```python
from build123d import *

# Parameters (mm, degrees)
F0_R     = 3
F1_DEPTH = 25
F2_DEPTH = 2
F3_DEPTH = 15
F4_SIZE2 = 1
F4_SIZE  = 2
F5_SIZE2 = 2
F5_SIZE  = 1


with BuildPart() as f1:
    # F0 (on Front) → F1 (new body)
    with BuildSketch(Plane.XZ):
        Circle(F0_R)
    extrude(amount=F1_DEPTH)

    # F0 (on Front) → F2 (join)
    with BuildSketch(Plane.XZ):
        with BuildLine():
            ThreePointArc((1.9364916731, -3.5), (3.4457195687, -2.0315060063), (4, 0))
            ThreePointArc((4, 0), (-2.0315060063, 3.4457195687), (-1.9364916731, -3.5))
            Line((-1.9364916731, -3.5), (1.9364916731, -3.5))
        make_face()
        Circle(F0_R, mode=Mode.SUBTRACT)
    extrude(amount=F2_DEPTH)

    # F0 (on Front) → F3 (join)
    with BuildSketch(Plane.XZ):
        Circle(F0_R)
    extrude(amount=-F3_DEPTH)

    # F4
    f4_edges = [f1.edges().sort_by_distance(p)[0] for p in [
        (-3, 15, 0),
    ]]
    f4_side = f1.faces().sort_by_distance((-3, 7.5, 0))[0]
    chamfer(f4_edges, length=F4_SIZE, length2=F4_SIZE2, reference=f4_side)

    # F5
    f5_edges = [f1.edges().sort_by_distance(p)[0] for p in [
        (-3, -25, 0),
    ]]
    f5_side = f1.faces().sort_by_distance((0, -25, 0))[0]
    chamfer(f5_edges, length=F5_SIZE, length2=F5_SIZE2, reference=f5_side)


solid = f1.part
```
The listing builds one solid part. Answer for the finished solid, in the listing's coordinates (mm). A direction names the side the tool comes from. Give positions to 0.01 mm unless a question says otherwise; leave off trailing zeros. Order: outer loops, then holes, each group sorted by start corner. A loop starts at its lowest first (then second) coordinate and runs counter-clockwise, first axis right, second up. Notation, with made-up numbers: (49.25, -18) - (63.25, -18) arc R16 ccw to (63.25, 4) - close; hole circle Ø7 at (-3, 14). An arc over 180 degrees is marked (long way). Answer in a Markdown table with one row per item. Add a question column.
Q1. The part is cut by section B-B (y = 12.5). Determine the outline of the cut face in (x, z), then the cut area to 3 significant figures.
Q2. Find the intervals of material crossed by line 1 along Y through (x, z) = (-3, 1); line 2 along Z through (x, y) = (0.25, -21); line 3 along X through (y, z) = (-6.5, -1.25), in increasing order. Write a range as [from, to].
Q3. The part is cut by section A-A (x = 0). Determine the outline of the cut face in (y, z), then the cut area to 3 significant figures.
Q4. Which of the six approach directions +Z, -Z, +X, -X, +Y, -Y give full straight-line access (tool end or side, diameter ignored) to faces 1 (the flat face through (1, 0, 3)), 2 (the flat face through (1, -2, 3)), 3 (the flat face through (0, 15, 0))?
Q5. Given P1, Ø1, axis at x = 2.5, z = -2.5, coming from the +Y side; P2, Ø1, axis at x = -0.5, y = -18, coming from the +Z side; P3, Ø1, axis at x = 2.5, y = -10.5, coming from the -Z side, each flat-ended and moving along its own axis, determine where each tip first touches the part or whether it passes through.
Determined:
| question | item | result |
|---|---|---|
| 1 | outline | circle Ø6 at (0, 0) |
| 1 | area | 28.3 mm² |
| 2 | line 1 | y = [-2, 0] |
| 2 | line 2 | z = [-2.99, 2.99] |
| 2 | line 3 | x = [-2.73, 2.73] |
| 3 | outline | (-25, -2) - (-23, -3) - (-2, -3) - (-2, -3.5) - (0, -3.5) - (0, -3) - (13, -3) - (15, -2) - (15, 2) - (13, 3) - (0, 3) - (0, 4) - (-2, 4) - (-2, 3) - (-23, 3) - (-25, 2) - close |
| 3 | area | 239 mm² |
| 4 | face 1 | +Y |
| 4 | face 2 | -Y |
| 4 | face 3 | +Z, -Z, +X, -X, +Y |
| 5 | P1 | stops at y = 0 |
| 5 | P2 | stops at z = 3 |
| 5 | P3 | stops at z = -2.24 |
